The listing builds one solid part. Answer for the finished solid, in the listing's coordinates (mm). A direction names the side the tool comes from. Give positions to 0.01 mm unless a question says otherwise; leave off trailing zeros. Write each loop counter-clockwise with the first axis right and the second up, starting at its lowest first coordinate (ties: lowest second). Pieces come first, ordered by that corner, then holes. Notation, with made-up numbers: (-29.75, -7.75) - (-9.75, -7.75) arc R10 ccw to (-9.75, 11.25) - close; hole circle Ø5 at (22, 0.5). An arc over 180 degrees is marked (long way). Write each question's results on one line, items separated by ' | '. Start each with the question number.
Q1. Find the intervals of material crossed by probe 1 along X at (y, z) = (-69, 48.5); probe 2 along X at (y, z) = (-87.5, 19); probe 3 along Z at (x, y) = (92, -69.75), in increasing order.
Q2. Section A-A (y = -82.5) is taken. Determine the outline of the cut face in (x, z), plus the area to 3 significant figures.
Q3. Section C-C (y = -72.25) is taken. Determine the outline of the cut face in (x, z), plus the area to 3 significant figures.
Q4. Section D-D (x = 88.5) is taken. Determine the outline of the cut face in (y, z), plus the area to 3 significant figures.
Q5. Section B-B (z = 17) is taken. Determine the outline of the cut face in (x, y).
Q6. For a pull along Y with two mould halves and no side action, classify faces 1 (the face through (96, -90.743, 31)), 2 (the face through (100.215, -78, 31)), 3 (the face through (91.464, -83.773, 30.776)), 4 (the face through (95, -64.468, 31)) as pulls with the +Y half, pulls with the -Y half, needs draft (parallel to the pull), parting line crosses it, or undercut.
Q7. Flat-ended cylindrical pins translate along their axes: pin 1 Ø6 at (y, z) = (-69, 19) entering from -X; pin 2 Ø6 at (y, z) = (-70, 30) entering from -X; pin 3 Ø1.8 at (x, y) = (89, -72) entering from +Z. Find the tip coordinate at first contact, or state that the pin passes through.
Q8. For faces 5 (the face through (92, -75, 47)), 6 (the face through (92, -75, 15)), 7 (the face through (88.71, -71.39, 30.78)), determine the directions among +Z, -Z, +X, -X, +Y, -Y from which every point of the face is accessible in a straight line to the end or side of a thin tool.
```python
from build123d import *

# Parameters (mm, degrees)
F1_DEPTH = 62
F3_W     = 26.2750325567
F3_H     = 15
F4_DEPTH = 25


with BuildPart() as f1:
    # F0 (on Top) → F1 (new body)
    with BuildSketch(Plane.XY):
        with BuildLine():
            Line((100.2154187574, -64.4678249955), (87.201975286, -64.4678249955))
            ThreePointArc((87.201975286, -64.4678249955), (88.7526881566, -71.4854053398), (93.1160420433, -77.1961222085))
            ThreePointArc((93.1160420433, -77.1961222085), (91.4511190136, -83.8686795317), (91.2494597241, -90.7428575522))
            Line((91.2494597241, -90.7428575522), (100.2154187574, -90.7428575522))
            Line((100.2154187574, -90.7428575522), (100.2154187574, -64.4678249955))
        make_face()
    extrude(amount=F1_DEPTH)

    # F3 (on offset) → F4 (cut)
    with BuildSketch(Plane.YZ.offset(93.2154187574)):
        with Locations((-77.6053412739, 54.5)):
            Rectangle(F3_W, F3_H)
        with Locations((-77.6053412739, 7.5)):
            Rectangle(F3_W, F3_H)
    extrude(amount=-F4_DEPTH, mode=Mode.SUBTRACT)


solid = f1.part
```
Answers below:
1) probe 1: x = 93.22 to 100.22 | probe 2: x = 91.16 to 100.22 | probe 3: z = 15 to 47
2) outline: (91.67, 15) - (93.22, 15) - (93.22, 0) - (100.22, 0) - (100.22, 62) - (93.22, 62) - (93.22, 47) - (91.67, 47) - close | area: 483 mm2
3) outline: (89.13, 15) - (93.22, 15) - (93.22, 0) - (100.22, 0) - (100.22, 62) - (93.22, 62) - (93.22, 47) - (89.13, 47) - close | area: 565 mm2
4) outline: (-70.91, 15) - (-64.47, 15) - (-64.47, 47) - (-70.91, 47) - close | area: 206 mm2
5) outline: (87.2, -64.47) arc R16.65 ccw to (93.12, -77.2) arc R32.02 ccw to (91.25, -90.74) - (100.22, -90.74) - (100.22, -64.47) - close
6) face 1: pulls with the -Y half | face 2: needs draft | face 3: undercut | face 4: pulls with the +Y half
7) pin 1: stops at x = 87.27 | pin 2: stops at x = 87.4 | pin 3: stops at z = 47
8) face 5: +Z, -X, +Y, -Y | face 6: -Z, -X, +Y, -Y | face 7: +Z, -Z, -X
